Here's how the part is built. I have some questions about the finished solid (model axes, mm). A direction names the side the tool comes from. Round coordinates to 2 decimals unless told otherwise and drop trailing zeros. Order: outer loops, then holes, each group sorted by start corner. A loop starts at its lowest first (then second) coordinate and runs counter-clockwise, first axis right, second up. Notation, with made-up numbers: (47, 15.5) - (91, 15.5) arc R13 cw to (91, 38.5) - close; hole circle Ø7 at (12.25, 62). An arc over 180 degrees is marked (long way). One line per item, written item: value.
from build123d import *

# Parameters (mm, degrees)
SKETCH1_W           = 11.9
SKETCH1_H           = 35
SKETCH1_W_2         = 7.9
SKETCH1_H_2         = 7.9
BOSS_EXTRUDE1_DEPTH = 2.8
SKETCH2_W           = 11.9
SKETCH2_H           = 35
BOSS_EXTRUDE2_DEPTH = 4
SKETCH3_W           = 11.9
SKETCH3_H           = 35
BOSS_EXTRUDE3_DEPTH = 1.6
CUT_EXTRUDE1_DEPTH  = 7.3
CHAMFER1_SIZE       = 1


with BuildPart() as part:
    # Sketch1 → Boss-Extrude1 (new body)
    with BuildSketch(Plane(origin=(0, 0, 0), x_dir=(1, 0, 0), z_dir=(0, 1, 0))):
        with Locations((0, 9.15)):
            Rectangle(SKETCH1_W, SKETCH1_H)
        Rectangle(SKETCH1_W_2, SKETCH1_H_2, mode=Mode.SUBTRACT)
    extrude(amount=BOSS_EXTRUDE1_DEPTH)

    # Sketch2 → Boss-Extrude2 (add)
    with BuildSketch(Plane(origin=(0, 2.8, 0), x_dir=(1, 0, 0), z_dir=(0, 1, 0))):
        with Locations((0, 9.15)):
            Rectangle(SKETCH2_W, SKETCH2_H)
        Polygon((-3.95, 3.95), (-3.45, 3.95), (-3.45, 24.65), (3.45, 24.65), (3.45, 3.95), (3.95, 3.95), (3.95, -3.95), (-3.95, -3.95), align=None, mode=Mode.SUBTRACT)
        Polygon((3.45, -3.45), (-3.45, -3.45), (-3.45, 3.45), (-3.45, 3.95), (-3.95, 3.95), (-3.95, -3.95), (3.95, -3.95), (3.95, 3.95), (3.45, 3.95), (3.45, 3.45), align=None)
    extrude(amount=BOSS_EXTRUDE2_DEPTH)

    # Sketch3 → Boss-Extrude3 (add)
    with BuildSketch(Plane(origin=(0, 6.8, 0), x_dir=(1, 0, 0), z_dir=(0, 1, 0))):
        with Locations((0, 9.15)):
            Rectangle(SKETCH3_W, SKETCH3_H)
    extrude(amount=BOSS_EXTRUDE3_DEPTH)

    # Sketch4 → Cut-Extrude1 (cut)
    with BuildSketch(Plane(origin=(0, -8.565144899, -3.117457795), x_dir=(-1, 0, 0), z_dir=(0, -0.9396926207859081, -0.34202014332566943))):
        with BuildLine():
            ThreePointArc((4.114090909, 18.618006757), (3.825, 18.917808344), (4.114090909, 19.217609931))
            ThreePointArc((4.114090909, 19.217609931), (2.916815472, 21.834623816), (0.299801587, 23.031899253))
            ThreePointArc((0.299801587, 23.031899253), (0, 22.742808344), (-0.299801587, 23.031899253))
            ThreePointArc((-0.299801587, 23.031899253), (-2.916815472, 21.834623816), (-4.114090909, 19.217609931))
            ThreePointArc((-4.114090909, 19.217609931), (-3.909045459, 19.126047717), (-3.825, 18.917808344))
            ThreePointArc((-3.825, 18.917808344), (-3.909045459, 18.709568971), (-4.114090909, 18.618006757))
            ThreePointArc((-4.114090909, 18.618006757), (-2.916815472, 16.000992872), (-0.299801587, 14.803717435))
            ThreePointArc((-0.299801587, 14.803717435), (0, 15.092808344), (0.299801587, 14.803717435))
            ThreePointArc((0.299801587, 14.803717435), (2.916815472, 16.000992872), (4.114090909, 18.618006757))
        make_face()
    extrude(amount=-CUT_EXTRUDE1_DEPTH, mode=Mode.SUBTRACT)

    # Chamfer1
    chamfer1_edges = [part.edges().sort_by_distance(p)[0] for p in [
        (0, 0, 3.95),
    ]]
    chamfer(chamfer1_edges, length=CHAMFER1_SIZE)


solid = part.part
Q1. If we section it at A-A, the plane z = -5: Please give me the cut outline in (x, y), then the cut area to 3 significant figures.
Results list:
outline: (-5.95, 0) - (5.95, 0) - (5.95, 8.4) - (-5.95, 8.4) - close; hole (-3.45, 2.8) - (3.45, 2.8) - (3.45, 6.8) - (-3.45, 6.8) - close
area: 72.4 mm²
Q2. If we section it at C-C, the plane z = 2: Please give me the cut outline in (x, y), then the cut area to 3 significant figures.
Results list:
outline: (-5.95, 0) - (-3.95, 0) - (-3.95, 2.8) - (-3.45, 2.8) - (-3.45, 6.8) - (3.45, 6.8) - (3.45, 2.8) - (3.95, 2.8) - (3.95, 0) - (5.95, 0) - (5.95, 8.4) - (-5.95, 8.4) - close
area: 50.2 mm²
Q3. Will this pin go through, and if not, where does the flat tip stop? pin 1 (2.5 mm diameter, centred on x = -0.5, z = -1.5, fed in from -Y).
Results list:
pin 1: y = 6.8
Q4. If we section it at D-D, the plane x = -0.75: Please give me the cut outline in (y, z).
Results list:
outline: (0, -26.65) - (8.4, -26.65) - (8.4, 8.35) - (0, 8.35) - (0, 4.95) - (1, 3.95) - (2.8, 3.95) - (2.8, 3.45) - (6.8, 3.45) - (6.8, -24.65) - (2.8, -24.65) - (2.8, -23.43) - (0, -24.45) - close; (0, -15.82) - (2.8, -14.8) - (2.8, -3.95) - (0, -3.95) - close
Q5. If I drill on line 1 along Z through (x, y) = (-0.5, 4.75); line 2 along X through (y, z) = (5.75, -6), over which ranges is the centre line in solid material (lowest first)?
Results list:
line 1: -26.65 to -24.65, 3.45 to 8.35
line 2: -5.95 to -3.45, 3.45 to 5.95
Q6. If we section it at B-B, the plane y = 6.25: Please give me the cut outline in (x, z).
Results list:
outline: (-5.95, -26.65) - (5.95, -26.65) - (5.95, 8.35) - (-5.95, 8.35) - close; hole (-3.45, -24.65) - (3.45, -24.65) - (3.45, 3.45) - (-3.45, 3.45) - close
Q7. Which directions (+Z, -Z, +X, -X, +Y, -Y) give clear straight access to the entire face, cutting with the end or side of a thin tool? Please do faces 1 (the flat face through (0, 0, -9)), 2 (the flat face through (0, 1, -3.95)), 3 (the cylindrical face through (2.9, 1.4, -16.5)).
Results list:
face 1: +Z, -Z, +X, -X, -Y
face 2: -Y
face 3: none
Q8. We'd pull the mould along Y, two halves only. Please class faces 4 (the flat face through (-0.06, 0.51, 4.44)), 5 (the flat face through (0, 4, 8.35)), 6 (the cylindrical face through (-3.364, 1.766, -22.029)): released by +Y, released by -Y, zero draft, split by the parting line, or undercut.
Results list:
face 4: released by -Y
face 5: zero draft
face 6: undercut
